The model under review builds one solid part; all positions refer to its coordinate system, in mm. A direction names the side the tool comes from. Give positions to 0.01 mm unless a question says otherwise; leave off trailing zeros. Order: outer loops, then holes, each group sorted by start corner. A loop starts at its lowest first (then second) coordinate and runs counter-clockwise, first axis right, second up.
```python
from build123d import *

# Parameters (mm, degrees)
F1_DEPTH = 19.05
F2_W     = 22.8103399277
F2_H     = 51.1389188468
F3_DEPTH = 38.1
F4_W     = 23.9186170459
F4_H     = 24.924851954
F5_DEPTH = 25.4
F7_D     = 44.45


with BuildPart() as f1:
    # F0 (on Top) → F1 (new body)
    with BuildSketch(Plane.XY):
        with BuildLine():
            Line((25.4, 38.1), (-63.5, 38.1))
            Line((-63.5, 38.1), (-63.5, -38.1))
            Line((-63.5, -38.1), (25.4, -38.1))
            ThreePointArc((25.4, -38.1), (52.3407683632, -26.9407683632), (63.5, 0))
            ThreePointArc((63.5, 0), (52.3407683632, 26.9407683632), (25.4, 38.1))
        make_face()
    extrude(amount=-F1_DEPTH)

    # F2 (on Front) → F3 (join, symmetric)
    with BuildSketch(Plane.XZ):
        with Locations((-52.2303506732, 25.5694594234)):
            Rectangle(F2_W, F2_H)
    extrude(amount=F3_DEPTH, both=True)

    # F4 (on face) → F5 (cut)
    with BuildSketch(Plane(origin=(-63.635520637, 0, 0), x_dir=(0, -1, 0), z_dir=(-1, 0, 0))):
        with Locations((26.1406914771, 38.6764928699)):
            Rectangle(F4_W, F4_H)
    extrude(amount=-F5_DEPTH, mode=Mode.SUBTRACT)

    # F7 (through all)
    with Locations(Plane.XY):
        with Locations((12.4624269083, 0)):
            Hole(F7_D / 2)


solid = f1.part
```
Item 1: Draft analysis for pull direction X (two halves, no side actions). For faces 4 (the flat face through (-52, -14.181, 39)), 5 (the cylindrical face through (-8.736, 6.676, -9.658)), 6 (the flat face through (-63.5, 1, -9)), state which applies: released by +X, released by -X, zero draft, split by the parting line, or undercut.
Values found:
face 4: zero draft
face 5: undercut
face 6: released by -X
Item 2: Clearance check with flat-ended pins moving along their axes: pin 1 Ø25 at (x, y) = (-55, -27.5) entering from +Z; pin 2 Ø21 at (y, z) = (-8, -12) entering from -X; pin 3 Ø2 at (x, y) = (8.5, 25.5) entering from +Z; pin 4 Ø5 at (x, z) = (9, 1) entering from -Y. State where each tip first meets the part, or that it passes through.
Values found:
pin 1: stops at z = 26.21
pin 2: stops at x = -63.5
pin 3: stops at z = 0
pin 4: stops at y = -38.1
Item 3: For line 1 (X direction, y = 20.5, z = 1.5); line 2 (Z direction, x = 42, y = 2); line 3 (Y direction, x = -51, z = 32), list the stretches that pass through material, from the lowest coordinate up.
Values found:
line 1: x = -63.64 to -40.83
line 2: z = -19.05 to 0
line 3: y = -14.18 to 38.1
Item 4: Take a section at A-A (y = -12). Give the boundary of the cut face in (x, z).
Values found:
outline: (-63.64, 0) - (-63.5, 0) - (-63.5, -19.05) - (-6.24, -19.05) - (-6.24, 0) - (-40.83, 0) - (-40.83, 51.14) - (-63.64, 51.14) - close; (31.17, -19.05) - (61.56, -19.05) - (61.56, 0) - (31.17, 0) - close
Item 5: For faces 1 (the flat face through (-52, -26, 26.214)), 2 (the flat face through (-63.636, 8, 25)), 3 (the flat face through (-40.825, 8, 25)), list the 3-axis set-ups (+Z, -Z, +X, -X, +Y, -Y) from which the entire face can be reached by the end or side of a thin tool; tool diameter is ignored.
Values found:
face 1: +Z, +X, -X, -Y
face 2: +Z, -Z, -X, +Y, -Y
face 3: +Z, +X, +Y, -Y
Item 6: Take a section at D-D (x = -15). Give the boundary of the cut face in (y, z), and give its area (3 significant figures).
Values found:
outline: (-38.1, -19.05) - (38.1, -19.05) - (38.1, 0) - (-38.1, 0) - close
area: 1,450 mm2
Item 7: Take a section at B-B (x = 30). Give the boundary of the cut face in (y, z).
Values found:
outline: (-37.82, -19.05) - (-13.65, -19.05) - (-13.65, 0) - (-37.82, 0) - close; (13.65, -19.05) - (37.82, -19.05) - (37.82, 0) - (13.65, 0) - close
Item 8: Take a section at C-C (z = 31.5). Give the boundary of the cut face in (x, y), and give its area (3 significant figures).
Values found:
outline: (-63.64, -14.18) - (-40.83, -14.18) - (-40.83, 38.1) - (-63.64, 38.1) - close
area: 1,190 mm2
